Check sheet for the modelled part. Datum: model origin and axes. Units: mm. Give positions to 0.01 mm unless a question says otherwise; leave off trailing zeros. Write each loop counter-clockwise with the first axis right and the second up, starting at its lowest first coordinate (ties: lowest second). Pieces come first, ordered by that corner, then holes. Notation, with made-up numbers: (12.5, 43.5) -> (66.5, 43.5) arc R13 ccw to (66.5, 50.5) -> close; hole circle Ø10 at (83, 56.25). An arc over 180 degrees is marked (long way). Write each question's results on one line, items separated by ' | '. Start each with the question number.
```python
from build123d import *

# Parameters (mm, degrees)
F0_R     = 6.35
F0_R_2   = 7.62
F1_DEPTH = 39.878
F2_R     = 5.08


with BuildPart() as f1:
    # F0 (on Front) → F1 (new body)
    with BuildSketch(Plane.XZ):
        Polygon((-254, -42.434722), (254, -42.434722), (254, 42.434722), (127, 42.434722), (-200.728908, 42.434722), (-254, 42.434722), align=None)
        with Locations((-200.728908, 0)):
            Circle(F0_R, mode=Mode.SUBTRACT)
        with Locations((127, 0)):
            Circle(F0_R_2, mode=Mode.SUBTRACT)
    extrude(amount=F1_DEPTH)

    # F2
    f2_edges = [f1.edges().sort_by_distance(p)[0] for p in [
        (0, 0, 42.434722),
        (0, 0, -42.434722),
        (119.38, 0, 0),
        (-207.078908, 0, 0),
        (0, -39.878, 42.434722),
        (0, -39.878, -42.434722),
        (-207.078908, -39.878, 0),
        (119.38, -39.878, 0),
    ]]
    fillet(f2_edges, radius=F2_R)


solid = f1.part
```
Item 1: Section check A-A on z = 0. Record the boundary of the cut face in (x, y).
Item 2: Mould release check, pull along X, two halves, no side actions. Record for faces 1 (the flat face through (4, -20, 42.435)), 2 (the flat face through (254, -20, -1)), 3 (the flat face through (-254, -20, 1)), 4 (the cylindrical face through (119.387, -19.731, 0.335)): pulls with the +X half, pulls with the -X half, needs draft (parallel to the pull), parting line crosses it, or undercut.
Item 3: Section check B-B on x = 127. Record the boundary of the cut face in (y, z), then the cut area to 3 significant figures.
Item 4: Thickness scan on probe 1 along Z at (x, y) = (127, -22); probe 2 along Z at (x, y) = (7.5, -37.5); probe 3 along Z at (x, y) = (198, -3.5). Record the ranges inside material, lowest first. Write a range as from..to.
Check sheet entries:
1) outline: (-254, -39.88) -> (-212.16, -39.88) arc R5.08 ccw to (-207.08, -34.8) -> (-207.08, -5.08) arc R5.08 ccw to (-212.16, 0) -> (-254, 0) -> close; (-194.38, -34.8) arc R5.08 ccw to (-189.3, -39.88) -> (114.3, -39.88) arc R5.08 ccw to (119.38, -34.8) -> (119.38, -5.08) arc R5.08 ccw to (114.3, 0) -> (-189.3, 0) arc R5.08 ccw to (-194.38, -5.08) -> close; (134.62, -34.8) arc R5.08 ccw to (139.7, -39.88) -> (254, -39.88) -> (254, 0) -> (139.7, 0) arc R5.08 ccw to (134.62, -5.08) -> close
2) face 1: needs draft | face 2: pulls with the +X half | face 3: pulls with the -X half | face 4: undercut
3) outline: (-39.88, -37.35) arc R5.08 ccw to (-34.8, -42.43) -> (-5.08, -42.43) arc R5.08 ccw to (0, -37.35) -> (0, -12.7) arc R5.08 ccw to (-5.08, -7.62) -> (-34.8, -7.62) arc R5.08 ccw to (-39.88, -12.7) -> close; (-39.88, 12.7) arc R5.08 ccw to (-34.8, 7.62) -> (-5.08, 7.62) arc R5.08 ccw to (0, 12.7) -> (0, 37.35) arc R5.08 ccw to (-5.08, 42.43) -> (-34.8, 42.43) arc R5.08 ccw to (-39.88, 37.35) -> close | area: 2,730 mm^2
4) probe 1: z = -42.43..-7.62, 7.62..42.43 | probe 2: z = -41.66..41.66 | probe 3: z = -42.18..42.18
